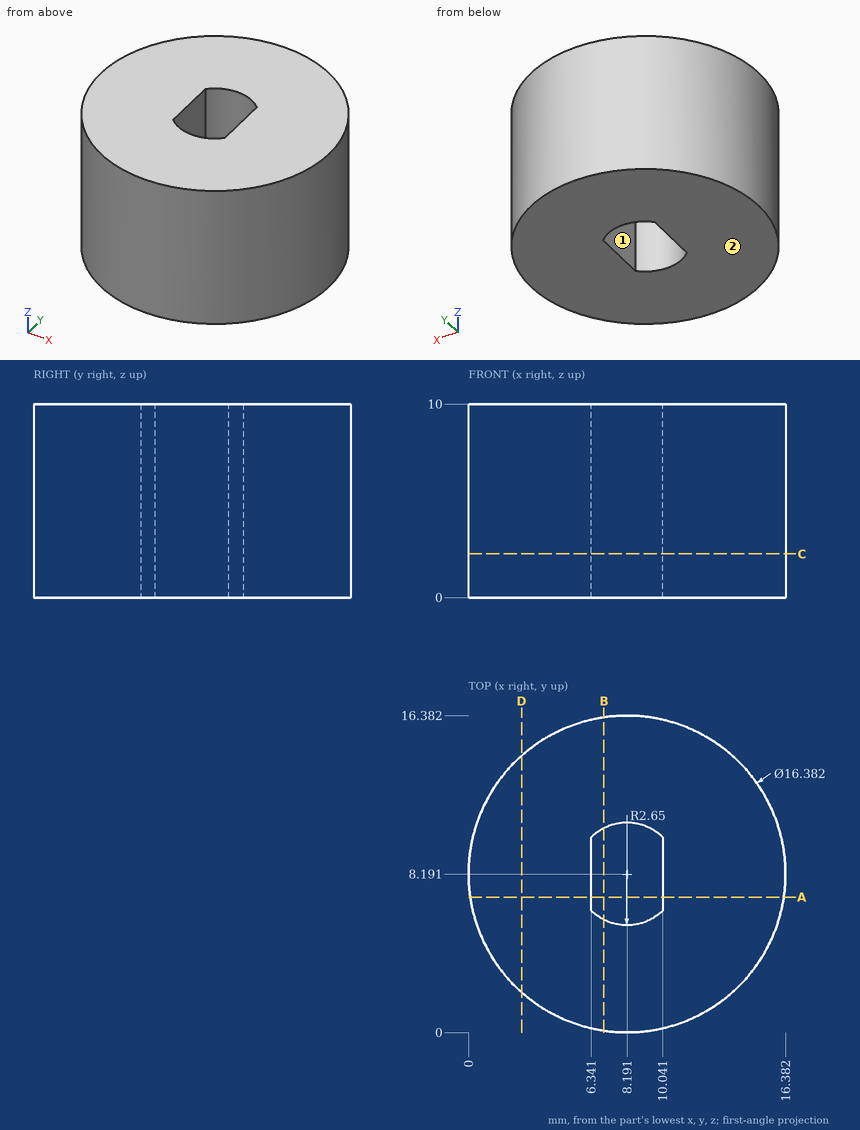
The figure shows three views and two pictorial views of one solid part (mm, origin at its lowest corner). Answer the questions. A direction names the side the tool comes from. Give positions to 0.01 mm unless a question says otherwise; leave off trailing zeros. Write each loop counter-clockwise with the first axis right and the second up, starting at its lowest first coordinate (ties: lowest second). Pieces come first, ordered by that corner, then holes. Notation, with made-up numbers: (-8.75, 82.25) -> (27.25, 82.25) arc R21 cw to (27.25, 100.25) -> close; hole circle Ø11 at (23, 15.25). An arc over 180 degrees is marked (long way). Use one line per item in the form item = value.
1) A tool of negligible diameter and unlimited length cuts with its end or side. For the marked faces 1 and 2, from which of +Z, -Z, +X, -X, +Y, -Y can it reach the whole face along a straight path? Write none if from no direction.
Result:
face_1 = +Z, -Z
face_2 = -Z, +X, -X, +Y, -Y
2) Section A-A on y = 7 is taken. Write down the section's boundary in (x, z) (3 decimals), plus the area to 3 significant figures.
Result:
outline = (0.087, 0) -> (6.341, 0) -> (6.341, 10) -> (0.087, 10) -> close; (10.041, 0) -> (16.295, 0) -> (16.295, 10) -> (10.041, 10) -> close
area = 125 mm²
3) Section C-C on z = 2.25 is taken. Write down the section's boundary in (x, y), plus the area to 3 significant figures.
Result:
outline = circle Ø16.38 at (8.19, 8.19); hole (6.34, 6.29) arc R2.65 ccw to (10.04, 6.29) -> (10.04, 10.09) arc R2.65 ccw to (6.34, 10.09) -> close
area = 193 mm²
4) Straight lines are drawn through the part: probe 1 along X at (y, z) = (8.5, 5.25); probe 2 along Y at (x, z) = (7.5, 7.25); probe 3 along Y at (x, z) = (7, 3.5) (3 decimals). For each, find the intervals that lie inside material, in ascending order.
Result:
probe_1 = 0.01 to 6.34, 10.04 to 16.38
probe_2 = 0.03 to 5.63, 10.75 to 16.35
probe_3 = 0.087 to 5.824, 10.558 to 16.295
5) Section B-B on x = 7 is taken. Write down the section's boundary in (y, z) (3 decimals).
Result:
outline = (0.087, 0) -> (5.824, 0) -> (5.824, 10) -> (0.087, 10) -> close; (10.558, 0) -> (16.295, 0) -> (16.295, 10) -> (10.558, 10) -> close
6) Section D-D on x = 2.75 is taken. Write down the section's boundary in (y, z), plus the area to 3 significant figures.
Result:
outline = (2.07, 0) -> (14.31, 0) -> (14.31, 10) -> (2.07, 10) -> close
area = 122 mm²
